from build123d import *

# Parameters (mm, degrees)
BOSS_EXTRUDE1_DEPTH = 15
SKETCH2_W           = 32.3
SKETCH2_H           = 2.5
BOSS_EXTRUDE2_DEPTH = 23.5
SKETCH3_W           = 5
SKETCH3_H           = 6.2
CUT_EXTRUDE1_DEPTH  = 12.5
CUT_EXTRUDE2_REACH  = 28
SKETCH4_R           = 3.45
SKETCH5_R           = 1.2
CUT_EXTRUDE3_DEPTH  = 2.5
CUT_EXTRUDE4_REACH  = 39.3
SKETCH6_R           = 1.55
FILLET2_R           = 2
SKETCH7_W           = 7.5
SKETCH7_H           = 7.5
SKETCH7_R           = 1.55
CUT_EXTRUDE5_DEPTH  = 1.5
CUT_EXTRUDE6_REACH  = 4.5
SKETCH8_RX          = 9.634046057
SKETCH8_RY          = 6.312870092
SKETCH8_W           = 10
SKETCH8_H           = 3.175


with BuildPart() as part:
    # Sketch1 → Boss-Extrude1 (new body)
    with BuildSketch(Plane(origin=(0, 0, 0), x_dir=(1, 0, 0), z_dir=(0, 1, 0))):
        Polygon((0, 29.994099724), (-26, 29.994099724), (-26, -7.305900276), (0, -7.305900276), (0, -0.005900276), (-2.5, -0.005900276), (-2.5, -4.805900276), (-23.5, -4.805900276), (-23.5, 27.494099724), (-2.5, 27.494099724), (-2.5, 22.694099724), (0, 22.694099724), align=None)
    extrude(amount=BOSS_EXTRUDE1_DEPTH)

    # Sketch2 → Boss-Extrude2 (add, through all)
    with BuildSketch(Plane(origin=(-23.5, 0, 0), x_dir=(0, 0, -1), z_dir=(1, 0, 0))):
        with Locations((11.344099724, 1.25)):
            Rectangle(SKETCH2_W, SKETCH2_H)
    extrude(amount=BOSS_EXTRUDE2_DEPTH)

    # Sketch3 → Cut-Extrude1 (cut)
    with BuildSketch(Plane(origin=(0, 0, -29.994099724), x_dir=(-1, 0, 0), z_dir=(0, 0, -1))):
        with Locations((16.375, 8.6)):
            Rectangle(SKETCH3_W, SKETCH3_H)
    extrude(amount=-CUT_EXTRUDE1_DEPTH, mode=Mode.SUBTRACT)

    # Sketch4 → Cut-Extrude2 (cut, up to next)
    with BuildSketch(Plane.ZY.offset(26), mode=Mode.PRIVATE) as cut_extrude2_sk1:
        with Locations((-16.544099724, 8.6)):
            Circle(SKETCH4_R)
    cut_extrude2_tool1 = extrude(cut_extrude2_sk1.sketch, amount=-CUT_EXTRUDE2_REACH, mode=Mode.PRIVATE) & part.part
    add(cut_extrude2_tool1.solids().sort_by_distance((-26, 8.6, -16.5441))[0], mode=Mode.SUBTRACT)

    # Sketch5 → Cut-Extrude3 (cut)
    with BuildSketch(Plane(origin=(0, 0, 0), x_dir=(0, 0, -1), z_dir=(1, 0, 0))):
        with Locations((-2.555900276, 8.6)):
            Circle(SKETCH5_R)
    cut_extrude3 = extrude(amount=-CUT_EXTRUDE3_DEPTH, mode=Mode.SUBTRACT)

    # Mirror1: Cut-Extrude3 across plane
    add(cut_extrude3.mirror(Plane.XY.offset(-11.344099724)), mode=Mode.SUBTRACT)

    # Sketch6 → Cut-Extrude4 (cut, up to next)
    with BuildSketch(Plane.XY.offset(7.305900276), mode=Mode.PRIVATE) as cut_extrude4_sk1:
        with Locations((-13, 8.75)):
            Circle(SKETCH6_R)
    cut_extrude4_tool1 = extrude(cut_extrude4_sk1.sketch, amount=-CUT_EXTRUDE4_REACH, mode=Mode.PRIVATE) & part.part
    add(cut_extrude4_tool1.solids().sort_by_distance((-13, 8.75, 7.3059))[0], mode=Mode.SUBTRACT)

    # Fillet2
    fillet2_edges = [part.edges().sort_by_distance(p)[0] for p in [
        (0, 0, -11.344099724),
        (-13, 0, 7.305900276),
        (-26, 0, -11.344099724),
        (-13, 0, -29.994099724),
        (0, 7.5, 7.305900276),
        (-26, 7.5, 7.305900276),
        (-26, 7.5, -29.994099724),
        (0, 7.5, -29.994099724),
    ]]
    fillet(fillet2_edges, radius=FILLET2_R)

    # Sketch7 → Cut-Extrude5 (cut)
    with BuildSketch(Plane.XY.offset(7.305900276)):
        with Locations((-13, 8.75)):
            Rectangle(SKETCH7_W, SKETCH7_H)
        with Locations((-13, 8.75)):
            Circle(SKETCH7_R, mode=Mode.SUBTRACT)
    extrude(amount=-CUT_EXTRUDE5_DEPTH, mode=Mode.SUBTRACT)

    # Sketch8 → Cut-Extrude6 (cut, up to next)
    with BuildSketch(Plane(origin=(0, 2.5, 0), x_dir=(1, 0, 0), z_dir=(0, 1, 0)), mode=Mode.PRIVATE) as cut_extrude6_sk1:
        with Locations(Location((-13, 11.344099724), (0, 0, 90))):
            Ellipse(SKETCH8_RX, SKETCH8_RY)
    cut_extrude6_tool1 = extrude(cut_extrude6_sk1.sketch, amount=-CUT_EXTRUDE6_REACH, mode=Mode.PRIVATE) & part.part
    add(cut_extrude6_tool1.solids().sort_by_distance((-13, 2.5, -11.3441))[0], mode=Mode.SUBTRACT)
    # Sketch8 → Cut-Extrude6 (cut, up to next)
    with BuildSketch(Plane(origin=(0, 2.5, 0), x_dir=(1, 0, 0), z_dir=(0, 1, 0)), mode=Mode.PRIVATE) as cut_extrude6_sk2:
        with Locations((-13, -2.231384095)):
            Rectangle(SKETCH8_W, SKETCH8_H)
    cut_extrude6_tool2 = extrude(cut_extrude6_sk2.sketch, amount=-CUT_EXTRUDE6_REACH, mode=Mode.PRIVATE) & part.part
    add(cut_extrude6_tool2.solids().sort_by_distance((-13, 2.5, 2.231384))[0], mode=Mode.SUBTRACT)
    # Sketch8 → Cut-Extrude6 (cut, up to next)
    with BuildSketch(Plane(origin=(0, 2.5, 0), x_dir=(1, 0, 0), z_dir=(0, 1, 0)), mode=Mode.PRIVATE) as cut_extrude6_sk3:
        with Locations((-13, 24.919583542)):
            Rectangle(SKETCH8_W, SKETCH8_H)
    cut_extrude6_tool3 = extrude(cut_extrude6_sk3.sketch, amount=-CUT_EXTRUDE6_REACH, mode=Mode.PRIVATE) & part.part
    add(cut_extrude6_tool3.solids().sort_by_distance((-13, 2.5, -24.919584))[0], mode=Mode.SUBTRACT)


solid = part.part
Source: CAD feature listing. Evaluate the final solid. Frame: model axes, mm. A direction names the side the tool comes from. Round coordinates to 2 decimals unless told otherwise and drop trailing zeros. Order: outer loops, then holes, each group sorted by start corner. A loop starts at its lowest first (then second) coordinate and runs counter-clockwise, first axis right, second up. Notation, with made-up numbers: (-2, 58) - (9, 58) arc R38 cw to (9, 96) - close; hole circle Ø1 at (-30.5, 49). An arc over 180 degrees is marked (long way). Use a Markdown table: item, result. Add a question column.
1. Section query A-A (y = 13.25). Return the cut outline in (x, z).
2. Section query B-B (x = -20.25). Return the cut outline in (y, z).
3. Mould query, pull axis X, two halves, no side actions, for faces 5 (the flat face through (-8, 1, -25)), 6 (the cylindrical face through (-12.846, 0.57, 6.704)), 7 (the flat face through (-26, 8, -12)). Classes: +X half, -X half, draft (parallel to the pull), parting line (faces both ways), or undercut.
4. Section query C-C (x = -13). Give the number of separate pieces and of enclosed holes in the cut face, then the cut area to 3 significant figures.
5. First-contact query: pin 1 (3 mm diameter, centred on x = -14, z = -17.5, fed in from -Y); pin 2 (0.8 mm diameter, centred on y = 8, z = 6.5, fed in from +X); pin 3 (3.5 mm diameter, centred on x = -13, y = 8.75, fed in from +Z); pin 4 (0.8 mm diameter, centred on y = 1, z = 2.5, fed in from +X). Flat tips, straight axial feed; report the tip coordinate or a pass-through.
6. Line query: probe 1 along Z at (x, y) = (-23.25, 9); probe 2 along Y at (x, z) = (-13, 5.3); probe 3 along X at (y, z) = (12, -27). Output: solid intervals per line, ascending.
7. Set-up query: faces 1 (the cylindrical face through (-1.23, 8.96, -24.1)), 2 (the flat face through (-13.1, 10.5, 5.806)), 3 (the flat face through (-13, 1, -23.332)), 4 (the flat face through (-2.5, 9, 1)). Return all of +Z, -Z, +X, -X, +Y, -Y with unobstructed straight access to the full face (end or side cutting, diameter ignored); none if empty.
Derived:
| question | item | result |
|---|---|---|
| 1 | outline | (-26, -27.99) arc R2 ccw to (-24, -29.99) - (-2, -29.99) arc R2 ccw to (0, -27.99) - (0, -22.69) - (-2.5, -22.69) - (-2.5, -27.49) - (-23.5, -27.49) - (-23.5, 4.81) - (-2.5, 4.81) - (-2.5, 0.01) - (0, 0.01) - (0, 5.31) arc R2 ccw to (-2, 7.31) - (-24, 7.31) arc R2 ccw to (-26, 5.31) - close |
| 2 | outline | (0, -27.99) arc R2 ccw to (2, -29.99) - (15, -29.99) - (15, -27.49) - (2.5, -27.49) - (2.5, 4.81) - (15, 4.81) - (15, 7.31) - (2, 7.31) arc R2 ccw to (0, 5.31) - close |
| 3 | face 5 | undercut |
| 3 | face 6 | draft |
| 3 | face 7 | -X half |
| 4 | separate pieces | 5 |
| 4 | enclosed holes | 0 |
| 4 | area | 75.6 mm2 |
| 5 | pin 1 | through |
| 5 | pin 2 | x = -0.16 |
| 5 | pin 3 | z = 5.81 |
| 5 | pin 4 | x = -0.09 |
| 6 | probe 1 | -29.99 to -27.49, 4.81 to 7.31 |
| 6 | probe 2 | 0 to 7.2, 10.3 to 15 |
| 6 | probe 3 | -26 to -23.5, -2.5 to 0 |
| 7 | face 1 | +X |
| 7 | face 2 | +Z |
| 7 | face 3 | +Y, -Y |
| 7 | face 4 | +Y |
